Could you check a few things on this model? Use its own coordinates, in mm. A direction names the side the tool comes from. Give positions to 0.01 mm unless a question says otherwise; leave off trailing zeros. Write each loop counter-clockwise with the first axis right and the second up, starting at its lowest first coordinate (ties: lowest second). Pieces come first, ordered by that corner, then holes. Notation, with made-up numbers: M 6.25,49 L 34.25,49 A30 cw 34.25,88 Z; hole C 1,58.5 d6. An arc over 180 degrees is marked long. Use one line per item in the form item = value.
from build123d import *

# Parameters (mm, degrees)
F0_W           = 170
F0_H           = 100
F1_DEPTH       = 15
F3_D           = 8.5
F3_CBORE_D     = 13.75
F3_CBORE_DEPTH = 10
F5_D           = 15
F7_D           = 14.5
F9_D           = 16.5
F9_CBORE_D     = 30.1
F9_CBORE_DEPTH = 7.5


with BuildPart() as f1:
    # F0 (on Top) → F1 (new body)
    with BuildSketch(Plane.XY):
        with Locations((85, 50)):
            Rectangle(F0_W, F0_H)
    extrude(amount=-F1_DEPTH)

    # F3 (through all)
    with Locations(Plane.XY):
        with Locations((22.5, 87.5), (22.5, 12.5), (147.5, 87.5), (147.5, 12.5)):
            CounterBoreHole(F3_D / 2, F3_CBORE_D / 2, F3_CBORE_DEPTH)

    # F5 (through all)
    with Locations(Plane.XY):
        with Locations((20, 50), (150, 50)):
            Hole(F5_D / 2)

    # F7 (through all)
    with Locations(Plane.XY):
        with Locations((65, 50), (85, 50)):
            Hole(F7_D / 2)

    # F9 (through all)
    with Locations(Plane.XY):
        with Locations((110, 50)):
            CounterBoreHole(F9_D / 2, F9_CBORE_D / 2, F9_CBORE_DEPTH)


solid = f1.part
1) I want a section at C-C, the plane x = 150. Please give me the cut outline in (y, z).
Checked values:
outline = M 0,-15 L 9.06,-15 L 9.06,-10 L 6.1,-10 L 6.1,0 L 0,0 Z; M 15.94,-15 L 42.5,-15 L 42.5,0 L 18.9,0 L 18.9,-10 L 15.94,-10 Z; M 57.5,-15 L 84.06,-15 L 84.06,-10 L 81.1,-10 L 81.1,0 L 57.5,0 Z; M 90.94,-15 L 100,-15 L 100,0 L 93.9,0 L 93.9,-10 L 90.94,-10 Z
2) I want a section at D-D, the plane y = 12.5. Please give me the cut outline in (x, z) (3 decimals), plus the area to 3 significant figures.
Checked values:
outline = M 0,-15 L 18.25,-15 L 18.25,-10 L 15.625,-10 L 15.625,0 L 0,0 Z; M 26.75,-15 L 143.25,-15 L 143.25,-10 L 140.625,-10 L 140.625,0 L 29.375,0 L 29.375,-10 L 26.75,-10 Z; M 151.75,-15 L 170,-15 L 170,0 L 154.375,0 L 154.375,-10 L 151.75,-10 Z
area = 2,190 mm2
3) For pin 1 Ø3 at (x, z) = (98.5, -11.5) entering from -Y; pin 2 Ø9 at (x, y) = (150, 50) entering from +Z; pin 3 Ø15 at (x, y) = (112.5, 56) entering from +Z, each with a flat end and sliding along its axis, tell me the tip position at first contact or that it passes through.
Checked values:
pin_1 = 0
pin_2 = through
pin_3 = -7.5
4) For faces 1 (the flat face through (27, 13, -10)), 2 (the cylindrical face through (21.63, 42.68, -7.6)), which set-ups out of +Z, -Z, +X, -X, +Y, -Y let a thin tool reach every point of the face, with its end or its side?
Checked values:
face_1 = +Z
face_2 = +Z, -Z
5) If I drill on L1, parallel to Y at x = 85, z = -11; L2, parallel to Y at x = 147.5, z = -13.35; L3, parallel to Y at x = 110, z = -3.75, over which ranges is the centre line in solid material (lowest first)?
Checked values:
L1 = 0 to 42.75, 57.25 to 100
L2 = 0 to 8.25, 16.75 to 42.93, 57.07 to 83.25, 91.75 to 100
L3 = 0 to 34.95, 65.05 to 100
6) I want a section at B-B, the plane z = -2. Count the separate pieces of the cut face and the enclosed holes in it, plus the area to 3 significant figures.
Checked values:
separate_pieces = 1
enclosed_holes = 9
area = 15,000 mm2
7) Thinking about a two-plate mould opening in Y: for faces 3 (the flat face through (84, 62, 0)), 4 (the cylindrical face through (70.753, 45.588, -7.605)), 5 (the flat face through (84, 100, -7)), which applies, released by +Y, released by -Y, zero draft, split by the parting line, or undercut?
Checked values:
face_3 = zero draft
face_4 = undercut
face_5 = released by +Y
8) I want a section at A-A, the plane y = 50. Please give me the cut outline in (x, z), plus the area to 3 significant figures.
Checked values:
outline = M 0,-15 L 12.5,-15 L 12.5,0 L 0,0 Z; M 27.5,-15 L 57.75,-15 L 57.75,0 L 27.5,0 Z; M 72.25,-15 L 77.75,-15 L 77.75,0 L 72.25,0 Z; M 92.25,-15 L 101.75,-15 L 101.75,-7.5 L 94.95,-7.5 L 94.95,0 L 92.25,0 Z; M 118.25,-15 L 142.5,-15 L 142.5,0 L 125.05,0 L 125.05,-7.5 L 118.25,-7.5 Z; M 157.5,-15 L 170,-15 L 170,0 L 157.5,0 Z
area = 1,320 mm2
